Autodesk Inventor part; units mm, degrees
ref_plane "YZ Plane" through (0, 0, 0) normal (1, 0, 0) x (0, 1, 0)
ref_plane "XZ Plane" through (0, 0, 0) normal (0, 1, 0) x (-1, 0, 0)
ref_plane "XY Plane" through (0, 0, 0) normal (0, 0, 1) x (1, 0, 0)
sketch "Sketch1" plane through (0, 0, 0) normal (0, 0, 1) x (1, 0, 0)
  circle A0 centre (0, 0) radius 11.5
  line L0 (-18, -21) -> (18, -21)
  line L1 (21, -18) -> (21, 18)
  line L2 (18, 21) -> (-18, 21)
  line L3 (-21, 18) -> (-21, -18)
  line L4 (-21, -21) -> (21, 21) construction
  line L5 (21, -21) -> (-21, 21) construction
  circle A1 centre (-15.5, 15.5) radius 1.875
  circle A2 centre (15.5, 15.5) radius 1.875
  circle A3 centre (15.5, -15.5) radius 1.875
  circle A4 centre (-15.5, -15.5) radius 1.875
  line L6 (-15.5, 15.5) -> (15.5, 15.5) construction
  line L7 (15.5, 15.5) -> (15.5, -15.5) construction
  line L8 (15.5, -15.5) -> (-15.5, -15.5) construction
  line L9 (-15.5, 15.5) -> (-15.5, -15.5) construction
  line L10 (-15.5, 15.5) -> (15.5, -15.5) construction
  line L11 (15.5, 15.5) -> (0, 0) construction
  circle A5 centre (-23, 4) radius 3.95
  circle A6 centre (23, 4) radius 3.95
  circle A7 centre (-23, 4) radius 11
  circle A8 centre (23, 4) radius 11
  line L12 (0, 126.4593) -> (0, -125.5407)
  line L13 (-111.8366, 0) -> (126.1634, 0)
  circle A9 centre (-48.8366, 35.9593) radius 2.0625
  circle A10 centre (-57.8366, 80.4593) radius 2.0625
  circle A11 centre (-66.8366, 35.9593) radius 2.0625
  circle A12 centre (-66.8366, 60.9593) radius 2.0625
  circle A13 centre (-48.8366, 60.9593) radius 2.0625
  circle A14 centre (63.1634, 35.9593) radius 2.0625
  circle A15 centre (72.1634, 80.4593) radius 2.0625
  circle A16 centre (81.1634, 35.9593) radius 2.0625
  circle A17 centre (81.1634, 60.9593) radius 2.0625
  circle A18 centre (63.1634, 60.9593) radius 2.0625
  circle A19 centre (-48.8366, -35.0407) radius 2.0625
  circle A20 centre (-57.8366, -79.5407) radius 2.0625
  circle A21 centre (-66.8366, -35.0407) radius 2.0625
  circle A22 centre (-66.8366, -60.0407) radius 2.0625
  circle A23 centre (-48.8366, -60.0407) radius 2.0625
  circle A24 centre (63.1634, -35.0407) radius 2.0625
  circle A25 centre (63.1634, -60.0407) radius 2.0625
  circle A26 centre (81.1634, -60.0407) radius 2.0625
  circle A27 centre (81.1634, -35.0407) radius 2.0625
  circle A28 centre (72.1634, -79.5407) radius 2.0625
  line L14 (92.1634, -89.5407) -> (92.1634, 90.4593)
  line L15 (92.1634, 90.4593) -> (-77.8366, 90.4593)
  line L16 (-77.8366, 90.4593) -> (-77.8366, -89.5407)
  line L17 (-77.8366, -89.5407) -> (92.1634, -89.5407)
  circle A29 centre (-48.8366, 35.9593) radius 2.0625
  circle A30 centre (-57.8366, 80.4593) radius 2.0625
  circle A31 centre (-66.8366, 35.9593) radius 2.0625
  circle A32 centre (-66.8366, 60.9593) radius 2.0625
  circle A33 centre (-48.8366, 60.9593) radius 2.0625
  circle A34 centre (63.1634, 35.9593) radius 2.0625
  circle A35 centre (72.1634, 80.4593) radius 2.0625
  circle A36 centre (81.1634, 35.9593) radius 2.0625
  circle A37 centre (81.1634, 60.9593) radius 2.0625
  circle A38 centre (63.1634, 60.9593) radius 2.0625
  circle A39 centre (-48.8366, -35.0407) radius 2.0625
  circle A40 centre (-57.8366, -79.5407) radius 2.0625
  circle A41 centre (-66.8366, -35.0407) radius 2.0625
  circle A42 centre (-66.8366, -60.0407) radius 2.0625
  circle A43 centre (-48.8366, -60.0407) radius 2.0625
  circle A44 centre (63.1634, -35.0407) radius 2.0625
  circle A45 centre (63.1634, -60.0407) radius 2.0625
  circle A46 centre (81.1634, -60.0407) radius 2.0625
  circle A47 centre (81.1634, -35.0407) radius 2.0625
  circle A48 centre (72.1634, -79.5407) radius 2.0625
  line L18 (92.1634, -89.5407) -> (92.1634, 90.4593)
  line L19 (92.1634, 90.4593) -> (-77.8366, 90.4593)
  line L20 (-77.8366, 90.4593) -> (-77.8366, -89.5407)
  line L21 (-77.8366, -89.5407) -> (92.1634, -89.5407)
  arc A49 (-18, 21) -> (-21, 18) centre (-18, 18) ccw
  arc A50 (21, 18) -> (18, 21) centre (18, 18) ccw
  arc A51 (18, -21) -> (21, -18) centre (18, -18) ccw
  arc A52 (-21, -18) -> (-18, -21) centre (-18, -18) ccw
  line L22 (-28.0915, -5.7507) -> (-21, -9.4536)
  line L23 (-28.0915, 13.7507) -> (-21, 17.4536)
  line L24 (28.0915, -5.7507) -> (21, -9.4536)
  line L25 (28.0915, 13.7507) -> (21, 17.4536)
  circle A53 centre (-23, 4) radius 5.5
  circle A54 centre (23, 4) radius 5.5
  dimension "d0" = 23
  dimension "d1" = 3.75
  dimension "d2" = 31
  dimension "d3" = 31
  dimension "d4" = 22
  dimension "d5" = 42
  dimension "d6" = 42
  dimension "d7" = 23
  dimension "d8" = 4
  dimension "d9" = 7.9
  dimension "d10" = 3
  dimension "d11" = 8
  dimension "d12" = 11
extrude "Extrusion1" add sketch "Sketch1" along normal blind 4 contours L13 A8 L1 A51 L0 L12 A0 | A0 L12 L2 A50 L1 A8 L13 | A0 L13 A7 L3 A49 L2 L12 | L12 L0 A52 L3 A7 L13 A0 | L13 A54 L1 A8 | A8 L1 A54 L13 | A8 L13 A54 L1 | L1 L25 A8 | A8 L24 L1 | L1 A54 L13 A8 | A54 L1 A6 L13 | L13 L1 A54 | L13 A53 L3 A7 | A7 L3 A53 L13 | A54 L13 L1 A6 | L1 L13 A54 | A7 L13 A53 L3 | L3 L22 A7 | A53 L3 L13 | L13 L3 A5 A53 | A6 L1 | L1 A6 | A53 L13 L3 | A7 L23 L3 | L3 A53 L13 A7 | L13 A53 L3 A5 | A5 L3 | L3 A5
sketch "Sketch2" plane through (0, 0, 4) normal (0, 0, 1) x (1, 0, 0)
  circle A0 centre (0, 0) radius 11.5
  circle A1 centre (-15.5, -15.5) radius 1.875
  circle A2 centre (15.5, -15.5) radius 1.875
  circle A3 centre (15.5, 15.5) radius 1.875
  circle A4 centre (-15.5, 15.5) radius 1.875
  line L0 (28.0915, 13.7507) -> (21, 17.4536)
  line L1 (21, 17.4536) -> (21, 18)
  arc A5 (21, 18) -> (18, 21) centre (18, 18) ccw
  line L2 (18, 21) -> (-18, 21)
  arc A6 (-18, 21) -> (-21, 18) centre (-18, 18) ccw
  line L3 (-21, 18) -> (-21, 17.4536)
  line L4 (-21, 17.4536) -> (-28.0915, 13.7507)
  arc A7 (-28.0915, 13.7507) -> (-28.0915, -5.7507) centre (-23, 4) ccw
  line L5 (-28.0915, -5.7507) -> (-21, -9.4536)
  line L6 (-21, -9.4536) -> (-21, -18)
  arc A8 (-21, -18) -> (-18, -21) centre (-18, -18) ccw
  line L7 (-18, -21) -> (18, -21)
  arc A9 (18, -21) -> (21, -18) centre (18, -18) ccw
  line L8 (21, -18) -> (21, -9.4536)
  line L9 (21, -9.4536) -> (28.0915, -5.7507)
  arc A10 (28.0915, -5.7507) -> (28.0915, 13.7507) centre (23, 4) ccw
  circle A11 centre (23, 4) radius 5.5
  circle A12 centre (-23, 4) radius 5.5
  circle A13 centre (23, 4) radius 3.95
  circle A14 centre (-23, 4) radius 3.95
  dimension "d15" = 11
  dimension "d16" = 7.9
  dimension "d17" = 7.9
  dimension "d18" = 11
extrude "Extrusion2" add sketch "Sketch2" along normal blind 8.5 contours A13 | A14
extrude "Extrusion3" add sketch "Sketch2" along normal blind 0.75 contours A11 | A12
fillet "Fillet1" radius 0.5 2 edges at (19.05, 4, 12.5) (-26.95, 4, 12.5)
sketch "Sketch3" plane through (23, 4, 12.5) normal (0, 0, 1) x (1, 0, 0)
  circle A0 centre (0, 0) radius 3.45
  circle A1 centre (-46, 0) radius 3.45
  circle A2 centre (0, 0) radius 2
  circle A3 centre (-46, 0) radius 2
  point P0 (-23, -4)
  dimension "d24" = 4
extrude "Extrusion4" cut sketch "Sketch3" against normal blind 8 contours A2 | A3
chamfer "Chamfer1" distance 0.25 angle 45 1 edges at (-26.95, 4, 4.75)
chamfer "Chamfer2" distance 0.25 angle 45 1 edges at (19.05, 4, 4.75)
properties part number "Stepper Atachments"
Model file for the job. Use its own axes, mm. A direction names the side the tool comes from. Coordinates: 2 decimals unless noted, no trailing zeros. Order: outer loops, then holes, each group sorted by start corner. A loop starts at its lowest first (then second) coordinate and runs counter-clockwise, first axis right, second up. Notation, with made-up numbers: (57, 66.5) -> (72, 66.5) arc R7 cw to (72, 79.5) -> close; hole circle Ø2 at (12.25, -36.5). An arc over 180 degrees is marked (long way). Return JSON: item names as keys, results as strings. Group by question number.
Item 1: Saw through at D-D on x = 23. Write the cut outline in (y, z), then the cut area to 3 significant figures.
Item 2: Saw through at A-A on x = 15.5. Write the cut outline in (y, z) (3 decimals).
Item 3: Wall check: line 1 along Y through (x, z) = (15.5, 1.95) (3 decimals); line 2 along X through (y, z) = (4.5, 11.75); line 3 along Y through (x, z) = (-7.5, 1.25). Give the ranges that are in metal, low to high. Write a range as [from, to].
Item 4: Tool access for faces 1 (the cylindrical face through (-1.5, -11.4, 2)), 2 (the flat face through (-21, -14, 2)), 3 (the cylindrical face through (-24.6, 2.8, 8.6)): list every direction of +Z, -Z, +X, -X, +Y, -Y with a clear straight run to the whole face (end or side of a thin tool).
Item 5: Saw through at C-C on z = 7.25. Write the cut outline in (x, y), then the cut area to 3 significant figures.
Item 6: Pull direction X, two halves, no side cores. Call faces 4 (the cylindrical face through (-19.232, 2.814, 8.451)), 5 (the flat face through (24.595, 15.576, 1.972)), 6 (the cylindrical face through (-20.14, 20.1, 1.97)): pulls with the +X half, pulls with the -X half, needs draft (parallel to the pull), parting line crosses it, or undercut.
Item 7: Flat gauge pins, fed straight in: P1, Ø12, axis at x = -25, y = -6.5, coming from the +Z side; P2, Ø12, axis at x = -14, y = 5.5, coming from the -Z side; P3, Ø1.2, axis at y = -14.5, z = 2.5, coming from the -X side; P4, Ø5, axis at x = -21.5, y = -2, coming from the +Z side. Where does each tip first touch, or does it go through?
Values found:
{
 "1": {"outline": "(-8.41, 0) -> (16.41, 0) -> (16.41, 4) -> (9.5, 4) -> (9.5, 4.75) -> (8.2, 4.75) -> (7.95, 5) -> (7.95, 12) arc R0.5 ccw to (7.45, 12.5) -> (6, 12.5) -> (6, 4.5) -> (2, 4.5) -> (2, 12.5) -> (0.55, 12.5) arc R0.5 ccw to (0.05, 12) -> (0.05, 5) -> (-0.2, 4.75) -> (-1.5, 4.75) -> (-1.5, 4) -> (-8.41, 4) -> close", "area": "137 mm2"},
 "2": {"outline": "(-21, 0) -> (-17.375, 0) -> (-17.375, 4) -> (-21, 4) -> close; (-13.625, 0) -> (13.625, 0) -> (13.625, 4) -> (-13.625, 4) -> close; (17.375, 0) -> (21, 0) -> (21, 4) -> (17.375, 4) -> close"},
 "3": {"line 1": "y = [-21, -17.375], [-13.625, 13.625], [17.375, 21]", "line 2": "x = [-26.92, -24.94], [-21.06, -19.08], [19.08, 21.06], [24.94, 26.92]", "line 3": "y = [-21, -8.72], [8.72, 21]"},
 "4": {"face 1": "+Z, -Z", "face 2": "+Z, -Z, -X, -Y", "face 3": "+Z"},
 "5": {"outline": "circle Ø7.9 at (-23, 4); circle Ø7.9 at (23, 4); hole circle Ø4 at (-23, 4); hole circle Ø4 at (23, 4)", "area": "72.9 mm2"},
 "6": {"face 4": "undercut", "face 5": "pulls with the +X half", "face 6": "pulls with the -X half"},
 "7": {"P1": "stops at z = 4.75", "P2": "stops at z = 0", "P3": "stops at x = -21", "P4": "stops at z = 12.44"}
}
